Could you check a few things on this drawing? It's one solid part, dimensions in mm from its lowest x, y, z. A direction names the side the tool comes from. Give positions to 0.01 mm unless a question says otherwise; leave off trailing zeros. Loops run counter-clockwise (first coordinate to the right, second up) from the corner with the lowest first, then second, coordinate; pieces in that order, holes last. Notation, with made-up numbers: M 86.5,36.25 L 100.5,36.25 A38 cw 100.5,75.25 Z; hole C 23.5,64.25 d11. An arc over 180 degrees is marked long. Return JSON: item names as keys, results as strings. Group by question number.
1. Please list where these lines run through material, in increasing order: line 1 (Y direction, x = 20.75, z = 6.25); line 2 (Y direction, x = 22.75, z = 15.25); line 3 (X direction, y = 14.25, z = 12.5).
2. If we section it at C-C (x = 15): Write out the boundary of the cut face in (y, z) (1 decimal).
3. If we mould it in two halves opening along Y, with no side actions, what happens to the marked faces 1, 2, 3 and 4? For each: +Y half, -Y half, draft (parallel to the pull), parting line (faces both ways), or undercut.
4. If we section it at B-B (z = 12.5): Write out the boundary of the cut face in (x, y).
5. For pin 1 (3 mm diameter, centred on x = 5, y = 9, fed in from -Z); pin 2 (0.8 mm diameter, centred on x = 23, y = 6.5, fed in from +Z); pin 3 (3 mm diameter, centred on x = 3.5, y = 10, fed in from +Z), each with a flat end and sliding along its axis, tell me the tip position at first contact or that it passes through.
6. If we section it at D-D (y = 14): Write out the boundary of the cut face in (x, z).
7. If we section it at A-A (x = 12.5): Write out the boundary of the cut face in (y, z).
8. For the marked faces 5, 6 and 7, which set-ups out of +Z, -Z, +X, -X, +Y, -Y let a thin tool reach every point of the face, with its end or its side?
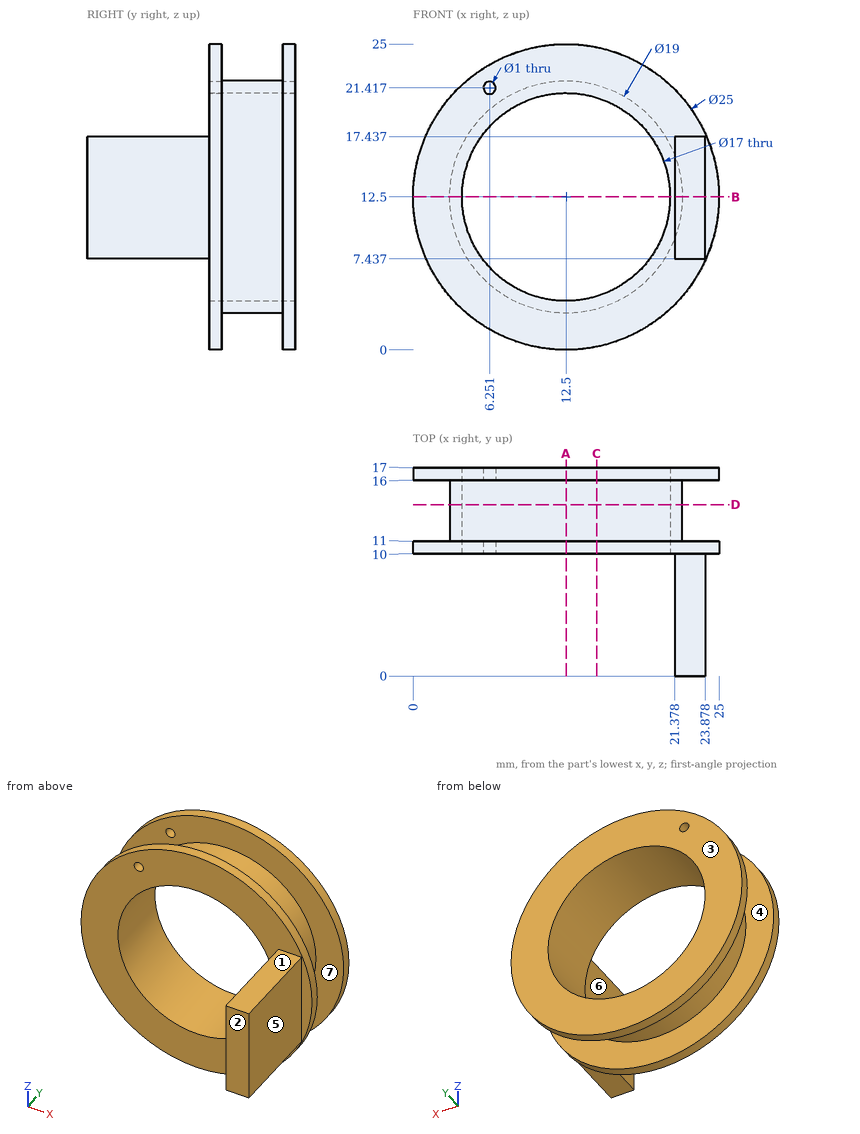
Answer:
{
 "1": {"line 1": "y = 10 to 11, 16 to 17", "line 2": "y = 0 to 11, 16 to 17", "line 3": "x = 3 to 4, 21 to 22"},
 "2": {"outline": "M 10,0.3 L 11,0.3 L 11,3.3 L 16,3.3 L 16,0.3 L 17,0.3 L 17,4.4 L 10,4.4 Z; M 10,20.6 L 17,20.6 L 17,24.7 L 16,24.7 L 16,21.7 L 11,21.7 L 11,24.7 L 10,24.7 Z"},
 "3": {"face 1": "draft", "face 2": "-Y half", "face 3": "+Y half", "face 4": "undercut"},
 "4": {"outline": "M 0,10 L 4,10 L 4,17 L 0,17 L 0,16 L 3,16 L 3,11 L 0,11 Z; M 21,10 L 21.38,10 L 21.38,0 L 23.88,0 L 23.88,10 L 25,10 L 25,11 L 22,11 L 22,16 L 25,16 L 25,17 L 21,17 Z"},
 "5": {"pin 1": "stops at z = 1.75", "pin 2": "stops at z = 17.44", "pin 3": "stops at z = 22.5"},
 "6": {"outline": "C 12.5,12.5 d19; hole C 12.5,12.5 d17"},
 "7": {"outline": "M 10,0 L 11,0 L 11,3 L 16,3 L 16,0 L 17,0 L 17,4 L 10,4 Z; M 10,21 L 17,21 L 17,25 L 16,25 L 16,22 L 11,22 L 11,25 L 10,25 Z"},
 "8": {"face 5": "+Z, -Z, +X, -Y", "face 6": "+Z, -Z, -X, -Y", "face 7": "none"}
}
